from build123d import *

# Parameters (mm, degrees)
EXTRUDE_1_DEPTH     = 1
CUT_EXTRUDE_1_REACH = 285.963
SKETCH_2_R          = 2.5


with BuildPart() as part:
    # Эскиз1 → Бобышка-Вытянуть1 (new body)
    with BuildSketch(Plane(origin=(0, 0, 0), x_dir=(0, 0, -1), z_dir=(1, 0, 0))):
        Polygon((223, -109.5), (223, 34.5), (262, 73.5), (262, 109.5), (-262, 109.5), (-262, -109.5), align=None)
    extrude(amount=EXTRUDE_1_DEPTH)

    # Эскиз2 → Вырез-Вытянуть1 (cut, up to next)
    with BuildSketch(Plane(origin=(1, 0, 0), x_dir=(0, 0, -1), z_dir=(1, 0, 0)), mode=Mode.PRIVATE) as cut_extrude_1_sk1:
        with Locations((40.5, -101.207106781)):
            Circle(SKETCH_2_R)
    cut_extrude_1_tool1 = extrude(cut_extrude_1_sk1.sketch, amount=-CUT_EXTRUDE_1_REACH, mode=Mode.PRIVATE) & part.part
    # Эскиз2 → Вырез-Вытянуть1 (cut, up to next)
    with BuildSketch(Plane(origin=(1, 0, 0), x_dir=(0, 0, -1), z_dir=(1, 0, 0)), mode=Mode.PRIVATE) as cut_extrude_1_sk2:
        with Locations((160.5, -101.207106781)):
            Circle(SKETCH_2_R)
    cut_extrude_1_tool2 = extrude(cut_extrude_1_sk2.sketch, amount=-CUT_EXTRUDE_1_REACH, mode=Mode.PRIVATE) & part.part
    # Эскиз2 → Вырез-Вытянуть1 (cut, up to next)
    with BuildSketch(Plane(origin=(1, 0, 0), x_dir=(0, 0, -1), z_dir=(1, 0, 0)), mode=Mode.PRIVATE) as cut_extrude_1_sk3:
        with Locations((-79.5, -101.207106781)):
            Circle(SKETCH_2_R)
    cut_extrude_1_tool3 = extrude(cut_extrude_1_sk3.sketch, amount=-CUT_EXTRUDE_1_REACH, mode=Mode.PRIVATE) & part.part
    # Эскиз2 → Вырез-Вытянуть1 (cut, up to next)
    with BuildSketch(Plane(origin=(1, 0, 0), x_dir=(0, 0, -1), z_dir=(1, 0, 0)), mode=Mode.PRIVATE) as cut_extrude_1_sk4:
        with Locations((-199.5, -101.207106781)):
            Circle(SKETCH_2_R)
    cut_extrude_1_tool4 = extrude(cut_extrude_1_sk4.sketch, amount=-CUT_EXTRUDE_1_REACH, mode=Mode.PRIVATE) & part.part
    # Эскиз2 → Вырез-Вытянуть1 (cut, up to next)
    with BuildSketch(Plane(origin=(1, 0, 0), x_dir=(0, 0, -1), z_dir=(1, 0, 0)), mode=Mode.PRIVATE) as cut_extrude_1_sk5:
        with Locations((215, -60.207106781)):
            Circle(SKETCH_2_R)
    cut_extrude_1_tool5 = extrude(cut_extrude_1_sk5.sketch, amount=-CUT_EXTRUDE_1_REACH, mode=Mode.PRIVATE) & part.part
    # Эскиз2 → Вырез-Вытянуть1 (cut, up to next)
    with BuildSketch(Plane(origin=(1, 0, 0), x_dir=(0, 0, -1), z_dir=(1, 0, 0)), mode=Mode.PRIVATE) as cut_extrude_1_sk6:
        with Locations((236.686291501, 59.792893219)):
            Circle(SKETCH_2_R)
    cut_extrude_1_tool6 = extrude(cut_extrude_1_sk6.sketch, amount=-CUT_EXTRUDE_1_REACH, mode=Mode.PRIVATE) & part.part
    # Эскиз2 → Вырез-Вытянуть1 (cut, up to next)
    with BuildSketch(Plane(origin=(1, 0, 0), x_dir=(0, 0, -1), z_dir=(1, 0, 0)), mode=Mode.PRIVATE) as cut_extrude_1_sk7:
        with Locations((-254, 59.792893219)):
            Circle(SKETCH_2_R)
    cut_extrude_1_tool7 = extrude(cut_extrude_1_sk7.sketch, amount=-CUT_EXTRUDE_1_REACH, mode=Mode.PRIVATE) & part.part
    # Эскиз2 → Вырез-Вытянуть1 (cut, up to next)
    with BuildSketch(Plane(origin=(1, 0, 0), x_dir=(0, 0, -1), z_dir=(1, 0, 0)), mode=Mode.PRIVATE) as cut_extrude_1_sk8:
        with Locations((-254, -60.207106781)):
            Circle(SKETCH_2_R)
    cut_extrude_1_tool8 = extrude(cut_extrude_1_sk8.sketch, amount=-CUT_EXTRUDE_1_REACH, mode=Mode.PRIVATE) & part.part
    # Эскиз2 → Вырез-Вытянуть1 (cut, up to next)
    with BuildSketch(Plane(origin=(1, 0, 0), x_dir=(0, 0, -1), z_dir=(1, 0, 0)), mode=Mode.PRIVATE) as cut_extrude_1_sk9:
        with Locations((-199.5, 100.5)):
            Circle(SKETCH_2_R)
    cut_extrude_1_tool9 = extrude(cut_extrude_1_sk9.sketch, amount=-CUT_EXTRUDE_1_REACH, mode=Mode.PRIVATE) & part.part
    # Эскиз2 → Вырез-Вытянуть1 (cut, up to next)
    with BuildSketch(Plane(origin=(1, 0, 0), x_dir=(0, 0, -1), z_dir=(1, 0, 0)), mode=Mode.PRIVATE) as cut_extrude_1_sk10:
        with Locations((-79.5, 100.5)):
            Circle(SKETCH_2_R)
    cut_extrude_1_tool10 = extrude(cut_extrude_1_sk10.sketch, amount=-CUT_EXTRUDE_1_REACH, mode=Mode.PRIVATE) & part.part
    # Эскиз2 → Вырез-Вытянуть1 (cut, up to next)
    with BuildSketch(Plane(origin=(1, 0, 0), x_dir=(0, 0, -1), z_dir=(1, 0, 0)), mode=Mode.PRIVATE) as cut_extrude_1_sk11:
        with Locations((40.5, 100.5)):
            Circle(SKETCH_2_R)
    cut_extrude_1_tool11 = extrude(cut_extrude_1_sk11.sketch, amount=-CUT_EXTRUDE_1_REACH, mode=Mode.PRIVATE) & part.part
    # Эскиз2 → Вырез-Вытянуть1 (cut, up to next)
    with BuildSketch(Plane(origin=(1, 0, 0), x_dir=(0, 0, -1), z_dir=(1, 0, 0)), mode=Mode.PRIVATE) as cut_extrude_1_sk12:
        with Locations((160.5, 100.5)):
            Circle(SKETCH_2_R)
    cut_extrude_1_tool12 = extrude(cut_extrude_1_sk12.sketch, amount=-CUT_EXTRUDE_1_REACH, mode=Mode.PRIVATE) & part.part
    add(cut_extrude_1_tool1.solids().sort_by_distance((1, -101.207107, -40.5))[0], mode=Mode.SUBTRACT)
    add(cut_extrude_1_tool2.solids().sort_by_distance((1, -101.207107, -160.5))[0], mode=Mode.SUBTRACT)
    add(cut_extrude_1_tool3.solids().sort_by_distance((1, -101.207107, 79.5))[0], mode=Mode.SUBTRACT)
    add(cut_extrude_1_tool4.solids().sort_by_distance((1, -101.207107, 199.5))[0], mode=Mode.SUBTRACT)
    add(cut_extrude_1_tool5.solids().sort_by_distance((1, -60.207107, -215))[0], mode=Mode.SUBTRACT)
    add(cut_extrude_1_tool6.solids().sort_by_distance((1, 59.792893, -236.686292))[0], mode=Mode.SUBTRACT)
    add(cut_extrude_1_tool7.solids().sort_by_distance((1, 59.792893, 254))[0], mode=Mode.SUBTRACT)
    add(cut_extrude_1_tool8.solids().sort_by_distance((1, -60.207107, 254))[0], mode=Mode.SUBTRACT)
    add(cut_extrude_1_tool9.solids().sort_by_distance((1, 100.5, 199.5))[0], mode=Mode.SUBTRACT)
    add(cut_extrude_1_tool10.solids().sort_by_distance((1, 100.5, 79.5))[0], mode=Mode.SUBTRACT)
    add(cut_extrude_1_tool11.solids().sort_by_distance((1, 100.5, -40.5))[0], mode=Mode.SUBTRACT)
    add(cut_extrude_1_tool12.solids().sort_by_distance((1, 100.5, -160.5))[0], mode=Mode.SUBTRACT)


solid = part.part
Model file for the job. Use its own axes, mm. Coordinates: 2 decimals unless noted, no trailing zeros. Write each loop counter-clockwise with the first axis right and the second up, starting at its lowest first coordinate (ties: lowest second). Pieces come first, ordered by that corner, then holes. Notation, with made-up numbers: (26, 53) -> (82, 53) arc R21 cw to (82, 74) -> close; hole circle Ø6 at (-7.75, -22.75). An arc over 180 degrees is marked (long way). One line per item, written item: value. Start each with the question number.
1) Probe probe 1 along Y at (x, z) = (0.75, 79.5); probe 2 along Z at (x, y) = (0.2, -59.5); probe 3 along Z at (x, y) = (0.4, 99.5). List the from-to ranges inside material, lowest first.
2) Slice it at B-B on y = 41. Write the cut outline in (x, z), then the cut area to 4 significant figures.
3) Slice it at C-C on y = 11. Write the cut outline in (x, z).
4) Slice it at A-A on x = 0.5. Count the separate pieces of the cut face and the enclosed holes in it, then the cut area to 3 significant figures.
Answers follow:
1. probe 1: -109.5 to -103.71, -98.71 to 98, 103 to 109.5
1. probe 2: -223 to -217.4, -212.6 to 251.6, 256.4 to 262
1. probe 3: -262 to -162.79, -158.21 to -42.79, -38.21 to 77.21, 81.79 to 197.21, 201.79 to 262
2. outline: (0, -229.5) -> (1, -229.5) -> (1, 262) -> (0, 262) -> close
2. area: 491.5 mm2
3. outline: (0, -223) -> (1, -223) -> (1, 262) -> (0, 262) -> close
4. separate pieces: 1
4. enclosed holes: 12
4. area: 108,000 mm2
